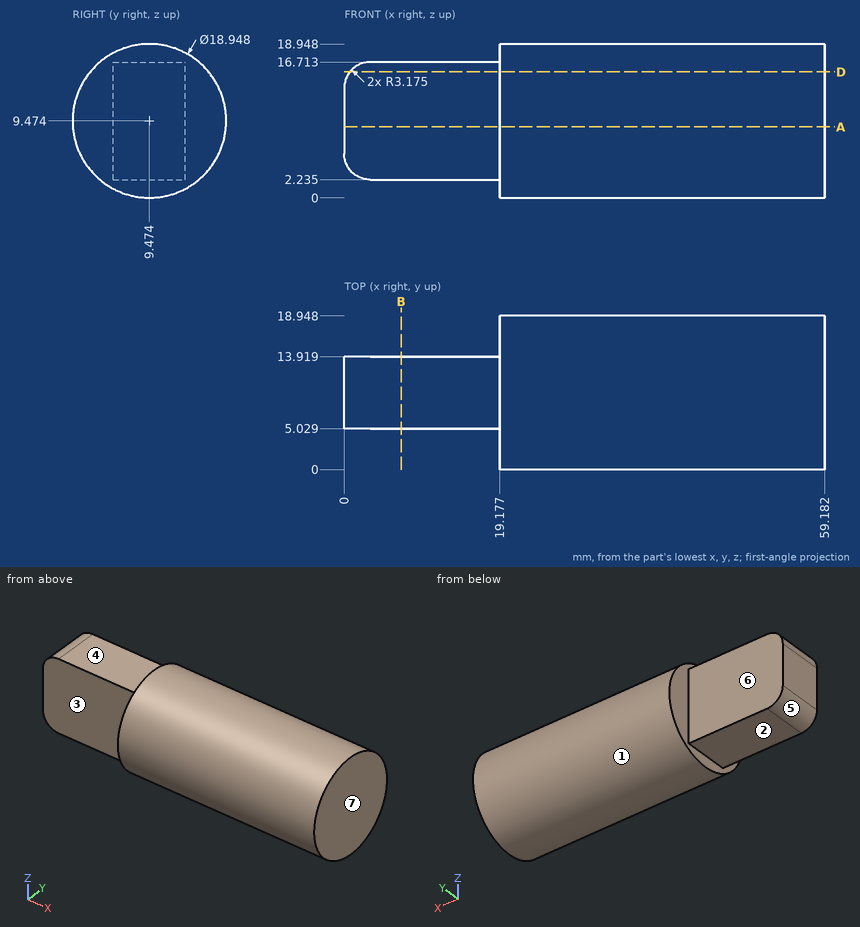
Part print with two shaded views. Sizes in mm from the minimum x, y, z corner. A direction names the side the tool comes from. Coordinates: 2 decimals unless noted, no trailing zeros. Order: outer loops, then holes, each group sorted by start corner. A loop starts at its lowest first (then second) coordinate and runs counter-clockwise, first axis right, second up. Notation, with made-up numbers: (3, -22) - (22, -22) arc R31 ccw to (22, 15) - close; hole circle Ø2 at (-15.75, 53). An arc over 180 degrees is marked (long way). Write item = value, one per line. Start each with the question number.
1) Wall check: line 1 along X through (y, z) = (4.75, 13.25); line 2 along Y through (x, z) = (22, 9.25) (1 decimal); line 3 along Y through (x, z) = (17, 16). Give the ranges that are in metal, low to high. Write a range as from..to.
2) Saw through at B-B on x = 7. Write the cut outline in (y, z) (1 decimal), then the cut area to 3 significant figures.
3) Flat gauge pins, fed straight in: pin 1 Ø2 at (x, y) = (29.5, 6.5) entering from +Z; pin 2 Ø2.5 at (x, y) = (8, 10) entering from +Z; pin 3 Ø10 at (x, y) = (12.5, 9) entering from -Z (1 decimal). Where does each tip first touch, or does it go through?
4) 3-axis set-ups, long thin cutter, end or side, ignore diameter. For the marked faces 1, 2, 3 and 4: which of +Z, -Z, +X, -X, +Y, -Y reach the whole face in a straight line?
5) Saw through at A-A on z = 8.75. Write the cut outline in (x, y), then the cut area to 3 significant figures.
6) Two-plate mould, pull along X, no slides. Class the marked faces 5, 6 and 7: pulls with the +X half, pulls with the -X half, needs draft (parallel to the pull), parting line crosses it, or undercut.
7) Saw through at D-D on z = 15.5. Write the cut outline in (x, y) (1 decimal).
From the geometry:
q1.line_1 = 19.18..59.18
q1.line_2 = 0..18.9
q1.line_3 = 5.03..13.92
q2.outline = (5, 2.2) - (13.9, 2.2) - (13.9, 16.7) - (5, 16.7) - close
q2.area = 129 mm^2
q3.pin_1 = 18.74
q3.pin_2 = 16.71
q3.pin_3 = 2.2
q4.face_1 = +X, -X
q4.face_2 = -Z, -X, +Y, -Y
q4.face_3 = +Z, -Z, -X, -Y
q4.face_4 = +Z, -X, +Y, -Y
q5.outline = (0, 5.03) - (19.18, 5.03) - (19.18, 0.03) - (59.18, 0.03) - (59.18, 18.92) - (19.18, 18.92) - (19.18, 13.92) - (0, 13.92) - close
q5.area = 926 mm^2
q6.face_5 = pulls with the -X half
q6.face_6 = needs draft
q6.face_7 = pulls with the +X half
q7.outline = (0.7, 5) - (19.2, 5) - (19.2, 2.2) - (59.2, 2.2) - (59.2, 16.8) - (19.2, 16.8) - (19.2, 13.9) - (0.7, 13.9) - close
